Geometry check sheet. Reference: the model listing, model coordinates, mm. A direction names the side the tool comes from. Round coordinates to 2 decimals unless told otherwise and drop trailing zeros. Loops run counter-clockwise (first coordinate to the right, second up) from the corner with the lowest first, then second, coordinate; pieces in that order, holes last. Notation, with made-up numbers: (4.25, 75.5) - (22.25, 75.5) arc R17 ccw to (22.25, 81.5) - close; hole circle Ø6 at (-26, 72). An arc over 180 degrees is marked (long way). Answer in a Markdown table with one row per item. Add a question column.
```python
from build123d import *

# Parameters (mm, degrees)
SKETCH1_W           = 38.1
SKETCH1_H           = 10.16
BOSS_EXTRUDE1_DEPTH = 127
SKETCH2_W           = 30.48
SKETCH2_H           = 7.112
CUT_EXTRUDE1_DEPTH  = 25.4
SKETCH3_R           = 7.239
CUT_EXTRUDE2_DEPTH  = 6.35
SKETCH4_R           = 5.207
CUT_EXTRUDE3_DEPTH  = 11.16
SKETCH5_R           = 8.641264269
BOSS_EXTRUDE2_DEPTH = 22.86
SKETCH6_R           = 7.239
CUT_EXTRUDE5_DEPTH  = 22.86


with BuildPart() as part:
    # Sketch1 → Boss-Extrude1 (new body)
    with BuildSketch(Plane.XY):
        Rectangle(SKETCH1_W, SKETCH1_H)
    extrude(amount=-BOSS_EXTRUDE1_DEPTH)

    # Sketch2 → Cut-Extrude1 (cut)
    with BuildSketch(Plane.XY):
        Rectangle(SKETCH2_W, SKETCH2_H)
    extrude(amount=-CUT_EXTRUDE1_DEPTH, mode=Mode.SUBTRACT)

    # Sketch3 → Cut-Extrude2 (cut)
    with BuildSketch(Plane(origin=(0, 5.08, 0), x_dir=(1, 0, 0), z_dir=(0, 1, 0))):
        with Locations((0, 118.618)):
            Circle(SKETCH3_R)
    extrude(amount=-CUT_EXTRUDE2_DEPTH, mode=Mode.SUBTRACT)

    # Sketch4 → Cut-Extrude3 (cut, through all)
    with BuildSketch(Plane.XZ.offset(5.08)):
        with Locations((0, -118.618)):
            Circle(SKETCH4_R)
    extrude(amount=-CUT_EXTRUDE3_DEPTH, mode=Mode.SUBTRACT)

    # Sketch5 → Boss-Extrude2 (add)
    with BuildSketch(Plane(origin=(0, 5.08, 0), x_dir=(1, 0, 0), z_dir=(0, 1, 0))):
        with Locations((0, 118.618)):
            Circle(SKETCH5_R)
    extrude(amount=BOSS_EXTRUDE2_DEPTH)

    # Sketch6 → Cut-Extrude5 (cut)
    with BuildSketch(Plane(origin=(0, 27.94, 0), x_dir=(1, 0, 0), z_dir=(0, 1, 0))):
        with Locations((0, 118.618)):
            Circle(SKETCH6_R)
    extrude(amount=-CUT_EXTRUDE5_DEPTH, mode=Mode.SUBTRACT)


solid = part.part
```
Q1. Cross-section at C-C, the plane z = -91. Enter the section's corners in (x, y), plus the area to 3 significant figures.
Q2. Cross-section at B-B, the plane y = 0. Enter the section's corners in (x, z).
Q3. Set-up check for faces 1 (the flat face through (-5, 27.94, -113)), 2 (the cylindrical face through (3.892, 13.539, -124.722)), 3 (the flat face through (0, 3.556, -13)): record each of +Z, -Z, +X, -X, +Y, -Y from which the full face is reachable in a straight line by a thin tool's end or side.
Q4. Cross-section at D-D, the plane y = 6.5. Enter the section's corners in (x, z).
Q5. Release check for a two-part mould opening along X. For faces 4 (the flat face through (0, 5.08, -63)), 5 (the flat face through (-19.05, 0, -63)), 6 (the flat face through (0, -3.556, -13)), 7 (the flat face through (19.05, 0, -63)) record: +X half, -X half, draft (parallel to the pull), parting line (faces both ways), or undercut.
Q6. Scan lines: line 1 (Y direction, x = 10.5, z = -14.5); line 2 (Z direction, x = 0, y = -3.3) (3 decimals); line 3 (Z direction, x = 0, y = 11). Record each from-to range of solid material in increasing order. Write a range as from..to.
Q7. Cross-section at A-A, the plane x = 0. Enter the section's corners in (y, z) (3 decimals).
Q8. Depth check by flat-ended pin: P1, Ø5, axis at x = -8, y = 1, coming from the -Z side; P2, Ø2, axis at x = -12, y = 0.5, coming from the +Z side; P3, Ø6, axis at x = -4, z = -77, coming from the +Y side. Enter the tip coordinate at first touch or a pass-through.
Check sheet entries:
| question | item | result |
|---|---|---|
| 1 | outline | (-19.05, -5.08) - (19.05, -5.08) - (19.05, 5.08) - (-19.05, 5.08) - close |
| 1 | area | 387 mm² |
| 2 | outline | (-19.05, -127) - (19.05, -127) - (19.05, 0) - (15.24, 0) - (15.24, -25.4) - (-15.24, -25.4) - (-15.24, 0) - (-19.05, 0) - close; hole circle Ø14.48 at (0, -118.62) |
| 3 | face 1 | +Z, -Z, +X, -X, +Y |
| 3 | face 2 | +Y |
| 3 | face 3 | +Z |
| 4 | outline | circle Ø17.28 at (0, -118.62); hole circle Ø14.48 at (0, -118.62) |
| 5 | face 4 | draft |
| 5 | face 5 | -X half |
| 5 | face 6 | undercut |
| 5 | face 7 | +X half |
| 6 | line 1 | -5.08..-3.56, 3.56..5.08 |
| 6 | line 2 | -127..-123.825, -113.411..-25.4 |
| 6 | line 3 | -127.26..-125.86, -111.38..-109.98 |
| 7 | outline | (-5.08, -127) - (5.08, -127) - (5.08, -127.259) - (27.94, -127.259) - (27.94, -125.857) - (-1.27, -125.857) - (-1.27, -123.825) - (-5.08, -123.825) - close; (-5.08, -113.411) - (-1.27, -113.411) - (-1.27, -111.379) - (27.94, -111.379) - (27.94, -109.977) - (5.08, -109.977) - (5.08, 0) - (3.556, 0) - (3.556, -25.4) - (-3.556, -25.4) - (-3.556, 0) - (-5.08, 0) - close |
| 8 | P1 | z = -127 |
| 8 | P2 | z = -25.4 |
| 8 | P3 | y = 5.08 |
